The listing builds one solid part. Answer for the finished solid, in the listing's coordinates (mm). Give positions to 0.01 mm unless a question says otherwise; leave off trailing zeros. Write each loop counter-clockwise with the first axis right and the second up, starting at its lowest first coordinate (ties: lowest second). Pieces come first, ordered by that corner, then holes. Notation, with made-up numbers: (-39.5, 80.25) - (-23.5, 80.25) arc R20 ccw to (-23.5, 93.25) - close; hole circle Ø9 at (71, 40.25). An arc over 180 degrees is marked (long way). One line per question, with ' | ' between items. Start each with the question number.
1. Given P1, Ø3, axis at x = 4.5, y = -6, coming from the -Z side; P2, Ø1, axis at x = 2, y = 11.5, coming from the -Z side, each flat-ended and moving along its own axis, determine where each tip first touches the part or whether it passes through.
2. Find the intervals of material crossed by L1, parallel to X at y = 9.5, z = 8.75 (3 decimals); L2, parallel to Y at x = 6, z = -4; L3, parallel to Y at x = 3.5, z = 3, in increasing order. Write a range as from..to.
3. A cutting plane is placed at D-D (x = 1.25). Determine the outline of the cut face in (y, z).
4. A cutting plane is placed at C-C (x = 5.25). Determine the outline of the cut face in (y, z) (1 decimal).
```python
from build123d import *

# Parameters (mm, degrees)
SKETCH1_R           = 12.6746
BOSS_EXTRUDE1_DEPTH = 3.175
SKETCH2_R           = 14.2875
BOSS_EXTRUDE2_DEPTH = 3.175


with BuildPart() as part:
    # Sketch1 → Boss-Extrude1 (new body)
    with BuildSketch(Plane(origin=(0, 0, 0), x_dir=(0, 0, -1), z_dir=(1, 0, 0))):
        Circle(SKETCH1_R)
    extrude(amount=BOSS_EXTRUDE1_DEPTH)

    # Sketch2 → Boss-Extrude2 (add)
    with BuildSketch(Plane(origin=(3.175, 0, 0), x_dir=(0, 0, -1), z_dir=(1, 0, 0))):
        Circle(SKETCH2_R)
    extrude(amount=BOSS_EXTRUDE2_DEPTH)

    # Sketch3 → Revolve1 (revolve)
    with BuildSketch(Plane.XY, mode=Mode.PRIVATE) as revolve1_sk:
        with BuildLine():
            Line((2.38125, 12.7), (2.38125, 11.90625))
            Line((2.38125, 11.90625), (0.79375, 11.90625))
            Line((0.79375, 11.90625), (0.79375, 12.7))
            ThreePointArc((0.79375, 12.7), (1.5875, 13.49375), (2.38125, 12.7))
        make_face()
    revolve(revolve1_sk.sketch.rotate(Axis((0, 0, 0), (-1, 0, 0)), 90), axis=Axis((0, 0, 0), (-1, 0, 0)))


solid = part.part
```
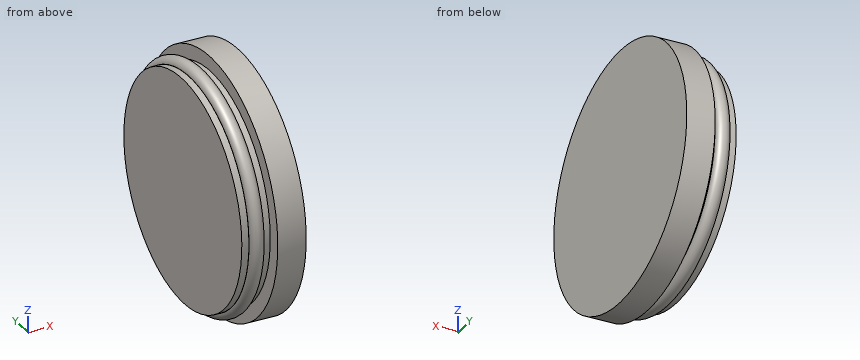
Determined:
1) P1: z = -13.56 | P2: z = -7.71
2) L1: 0.824..2.351, 3.175..6.35 | L2: -13.72..13.72 | L3: -13.97..13.97
3) outline: circle Ø26.84 at (0, 0)
4) outline: circle Ø28.6 at (0, 0)
